```python
from build123d import *

# Parameters (mm, degrees)
F1_DEPTH = 0.3
F3_D     = 5.5


with BuildPart() as f1:
    # F0 (on Front) → F1 (new body)
    with BuildSketch(Plane.XZ):
        with BuildLine():
            ThreePointArc((24.494897, -61), (32.267022, -49.558735), (35, -36))
            Line((35, -36), (35, -25.483315))
            Line((35, -25.483315), (35, -18))
            Line((35, -18), (35, -10.516685))
            Line((35, -10.516685), (35, 0))
            ThreePointArc((35, 0), (0, 35), (-35, 0))
            Line((-35, 0), (-35, -10.516685))
            Line((-35, -10.516685), (-35, -18))
            Line((-35, -18), (-35, -25.483315))
            Line((-35, -25.483315), (-35, -36))
            ThreePointArc((-35, -36), (-32.267022, -49.558735), (-24.494897, -61))
            ThreePointArc((-24.494897, -61), (0, -71), (24.494897, -61))
        make_face()
        with BuildLine():
            Line((-18, -25.183346), (-18, -10.816654))
            ThreePointArc((-18, -10.816654), (0, 21), (18, -10.816654))
            Line((18, -10.816654), (18, -25.183346))
            ThreePointArc((18, -25.183346), (0, -57), (-18, -25.183346))
        make_face(mode=Mode.SUBTRACT)
    extrude(amount=F1_DEPTH)

    # F3 (through all)
    with Locations(Plane.XZ.offset(0.3)):
        with Locations((0, 28.5), (-28.5, 0), (-28.5, -36), (0, -64.5), (28.5, -36), (28.5, 0)):
            Hole(F3_D / 2)


solid = f1.part
```
Verification items for the finished model (mm, model axes). Coordinates: 2 decimals unless noted, no trailing zeros. Order: outer loops, then holes, each group sorted by start corner. A loop starts at its lowest first (then second) coordinate and runs counter-clockwise, first axis right, second up. Notation, with made-up numbers: (41, 40.5) - (96, 40.5) arc R5 ccw to (96, 48.5) - close; hole circle Ø8 at (-32.75, 25.25). An arc over 180 degrees is marked (long way). Return JSON: item names as keys, results as strings.
(1) Section check A-A, the plane z = 11.5. Record the cut outline in (x, y), and give its area (3 significant figures).
Filled sheet:
{"outline": "(-33.06, -0.3) - (-17.57, -0.3) - (-17.57, 0) - (-33.06, 0) - close; (17.57, -0.3) - (33.06, -0.3) - (33.06, 0) - (17.57, 0) - close", "area": "9.29 mm^2"}
(2) Section check D-D, the plane x = 28.5. Record the cut outline in (y, z).
Filled sheet:
{"outline": "(-0.3, -56.32) - (0, -56.32) - (0, -38.75) - (-0.3, -38.75) - close; (-0.3, -33.25) - (0, -33.25) - (0, -2.75) - (-0.3, -2.75) - close; (-0.3, 2.75) - (0, 2.75) - (0, 20.32) - (-0.3, 20.32) - close"}
(3) Section check B-B, the plane x = 0. Record the cut outline in (y, z).
Filled sheet:
{"outline": "(-0.3, -71) - (0, -71) - (0, -67.25) - (-0.3, -67.25) - close; (-0.3, -61.75) - (0, -61.75) - (0, -57) - (-0.3, -57) - close; (-0.3, 21) - (0, 21) - (0, 25.75) - (-0.3, 25.75) - close; (-0.3, 31.25) - (0, 31.25) - (0, 35) - (-0.3, 35) - close"}
(4) Section check C-C, the plane y = -0.1. Record the cut outline in (x, z), and give its area (3 significant figures).
Filled sheet:
{"outline": "(-35, -36) arc R35 ccw to (-24.49, -61) arc R35 ccw to (24.49, -61) arc R35 ccw to (35, -36) - (35, 0) arc R35 ccw to (-35, 0) - close; hole circle Ø5.5 at (-28.5, -36); hole circle Ø5.5 at (-28.5, 0); hole (-18, -25.18) arc R21 ccw (long way) to (18, -25.18) - (18, -10.82) arc R21 ccw (long way) to (-18, -10.82) - close; hole circle Ø5.5 at (0, -64.5); hole circle Ø5.5 at (0, 28.5); hole circle Ø5.5 at (28.5, -36); hole circle Ø5.5 at (28.5, 0)", "area": "3,460 mm^2"}
(5) Thickness scan on line 1 along Z through (x, y) = (0, -0.1); line 2 along Z through (x, y) = (-2, -0.05); line 3 along Z through (x, y) = (-28.5, -0.1). Record the ranges inside material, lowest first.
Filled sheet:
{"line 1": "z = -71 to -67.25, -61.75 to -57, 21 to 25.75, 31.25 to 35", "line 2": "z = -70.94 to -66.39, -62.61 to -56.9, 20.9 to 26.61, 30.39 to 34.94", "line 3": "z = -56.32 to -38.75, -33.25 to -2.75, 2.75 to 20.32"}
(6) Go/stop test with flat-tipped pins: pin 1 (4.5 mm diameter, centred on x = 28.5, z = 0, fed in from +Y); pin 2 (4 mm diameter, centred on x = -24.5, z = -33.5, fed in from +Y). Record where each tip stops, or that it passes through.
Filled sheet:
{"pin 1": "passes through", "pin 2": "stops at y = 0"}
(7) Mould release check, pull along X, two halves, no side actions. Record for faces 1 (the flat face through (23, -0.3, -17)), 2 (the cylindrical face through (-31.12, -0.15, -35.17)): pulls with the +X half, pulls with the -X half, needs draft (parallel to the pull), parting line crosses it, or undercut.
Filled sheet:
{"face 1": "needs draft", "face 2": "undercut"}
